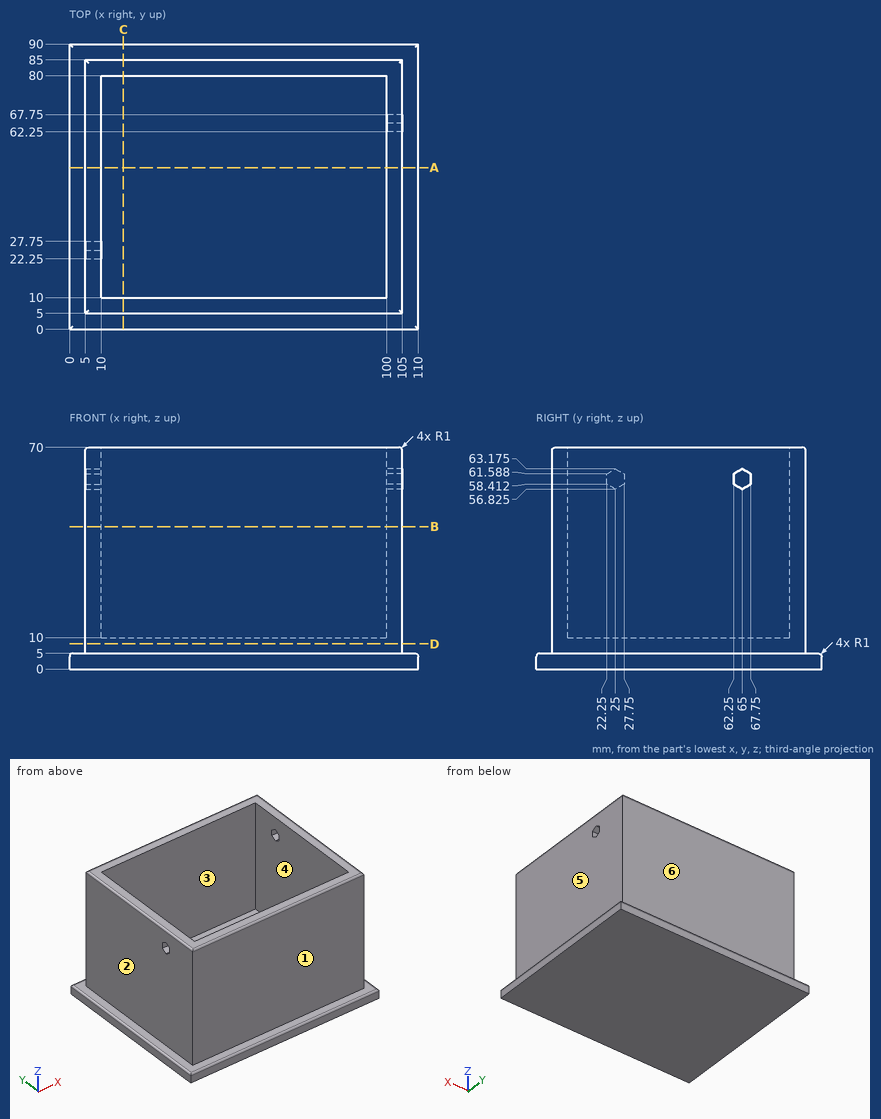
Part print with two shaded views. Sizes in mm from the minimum x, y, z corner. A direction names the side the tool comes from. Coordinates: 2 decimals unless noted, no trailing zeros. Write each loop counter-clockwise with the first axis right and the second up, starting at its lowest first coordinate (ties: lowest second). Pieces come first, ordered by that corner, then holes.
(1) Mould opens along Y. For the marked faces 4, 5 and 6 say: pulls with the +Y half, pulls with the -Y half, needs draft (parallel to the pull), parting line crosses it, or undercut.
(2) 3-axis set-ups, long thin cutter, end or side, ignore diameter. For the marked faces 1, 2 and 3: which of +Z, -Z, +X, -X, +Y, -Y reach the whole face in a straight line?
(3) Cut at A-A on y = 51. List the corners of the cut face in (x, z).
(4) Drill centre lines: line 1 (Y direction, x = 16, z = 12); line 2 (X direction, y = 16, z = 59.5); line 3 (Y direction, x = 10, z = 5.5). Where is each one in solid material? Low to high.
(5) Cut at C-C on x = 17. List the corners of the cut face in (y, z), and give its area (3 significant figures).
(6) Cut at D-D on z = 8. List the corners of the cut face in (x, y).
(7) Pin check, flat tips, straight feed: pin 1 Ø1.5 at (y, z) = (75, 44) entering from +X; pin 2 Ø2.5 at (x, z) = (8.5, 60.5) entering from -Y; pin 3 Ø4 at (x, y) = (24.5, 60.5) entering from +Z; pin 4 Ø4 at (x, y) = (89.5, 74) entering from -Z. Stop position of each tip, or through.
(8) Cut at B-B on z = 45. List the corners of the cut face in (x, y).
Working result:
1. face 4: undercut
1. face 5: needs draft
1. face 6: pulls with the +Y half
2. face 1: +Z, +X, -X, -Y
2. face 2: +Z, -X, +Y, -Y
2. face 3: +Z
3. outline: (0, 0) - (110, 0) - (110, 4) arc R1 ccw to (109, 5) - (105, 5) - (105, 69) arc R1 ccw to (104, 70) - (100, 70) - (100, 10) - (10, 10) - (10, 70) - (6, 70) arc R1 ccw to (5, 69) - (5, 5) - (1, 5) arc R1 ccw to (0, 4) - close
4. line 1: y = 5 to 10, 80 to 85
4. line 2: x = 5 to 10, 100 to 105
4. line 3: y = 5 to 85
5. outline: (0, 0) - (90, 0) - (90, 4) arc R1 ccw to (89, 5) - (85, 5) - (85, 69) arc R1 ccw to (84, 70) - (80, 70) - (80, 10) - (10, 10) - (10, 70) - (6, 70) arc R1 ccw to (5, 69) - (5, 5) - (1, 5) arc R1 ccw to (0, 4) - close
5. area: 1,450 mm2
6. outline: (5, 5) - (105, 5) - (105, 85) - (5, 85) - close
7. pin 1: stops at x = 105
7. pin 2: stops at y = 5
7. pin 3: stops at z = 10
7. pin 4: stops at z = 0
8. outline: (5, 5) - (105, 5) - (105, 85) - (5, 85) - close; hole (10, 10) - (100, 10) - (100, 80) - (10, 80) - close
